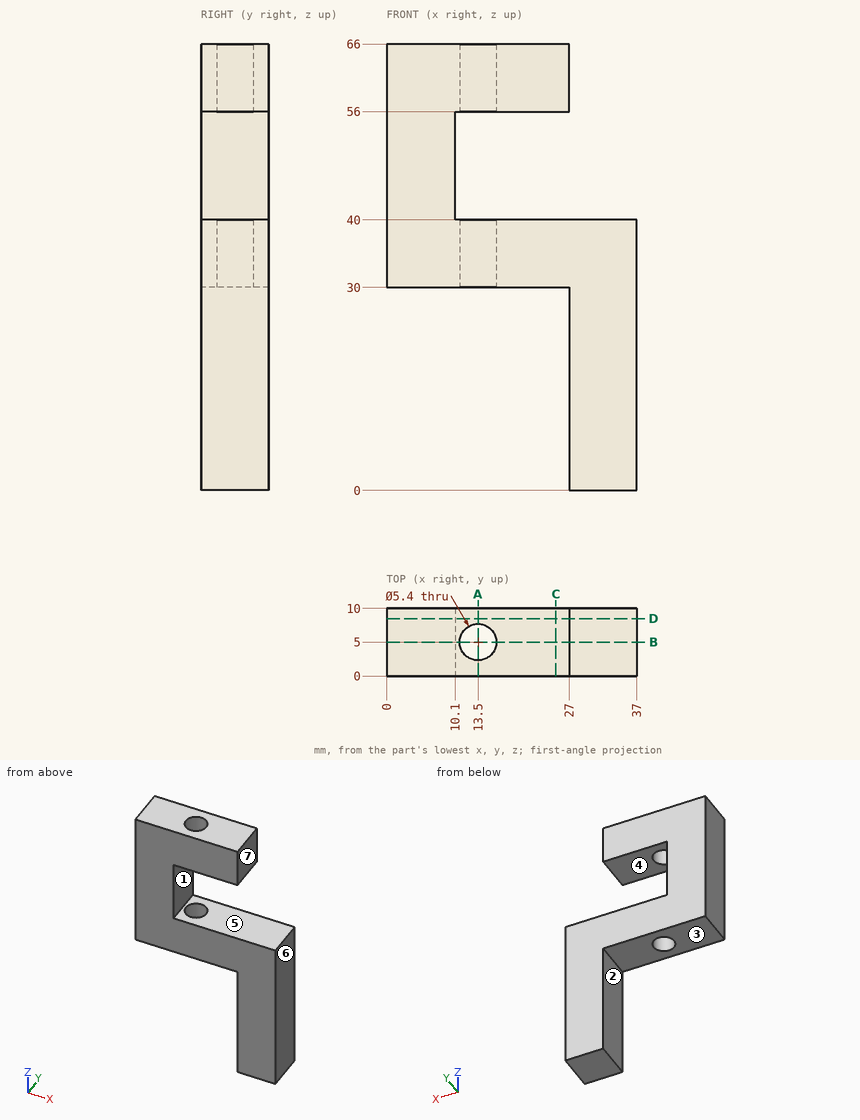
Design review of the part shown in the three views and the two pictorial views. Dimensions are in mm from the part's minimum x, y and z. A direction names the side the tool comes from. Coordinates: 2 decimals unless noted, no trailing zeros. Write each loop counter-clockwise with the first axis right and the second up, starting at its lowest first coordinate (ties: lowest second). Pieces come first, ordered by that corner, then holes.
1) We need section D-D on y = 8.5. State the section outline as (x, z) points.
2) We need section C-C on x = 25. State the section outline as (y, z) points.
3) We need section B-B on y = 5. State the section outline as (x, z) points, then the cut area to 3 significant figures.
4) The part is to be moulded in two halves that separate along Z. For the marked faces 1, 2, 3 and 4, say which applies: pulls with the +Z half, pulls with the -Z half, needs draft (parallel to the pull), parting line crosses it, or undercut.
5) To check wall thickness, follow probe 1 along Y at (x, z) = (13.5, 35.5); probe 2 along Z at (x, y) = (19.5, 8.5); probe 3 along X at (y, z) = (1.75, 19.5). State the ranges of each line that lie inside material, in increasing order.
6) Clearance check with flat-ended pins moving along their axes: pin 1 Ø3 at (x, y) = (13.5, 5) entering from -Z; pin 2 Ø1 at (x, y) = (7, 6) entering from -Z; pin 3 Ø1 at (y, z) = (5, 17.5) entering from -X. State where each tip first meets the part, or that it passes through.
7) We need section A-A on x = 13.5. State the section outline as (y, z) points.
8) Machinability: for the marked faces 5, 6 and 7, which of the approach directions +Z, -Z, +X, -X, +Y, -Y give a long, thin tool a straight path to every point of the face, cutting with its end or side? Answer none if there is none.
Answer list:
1. outline: (0, 30) - (27, 30) - (27, 0) - (37, 0) - (37, 40) - (10.1, 40) - (10.1, 56) - (27, 56) - (27, 66) - (0, 66) - close
2. outline: (0, 30) - (10, 30) - (10, 40) - (0, 40) - close; (0, 56) - (10, 56) - (10, 66) - (0, 66) - close
3. outline: (0, 30) - (10.8, 30) - (10.8, 40) - (10.1, 40) - (10.1, 56) - (10.8, 56) - (10.8, 66) - (0, 66) - close; (16.2, 30) - (27, 30) - (27, 0) - (37, 0) - (37, 40) - (16.2, 40) - close; (16.2, 56) - (27, 56) - (27, 66) - (16.2, 66) - close
3. area: 994 mm2
4. face 1: undercut
4. face 2: needs draft
4. face 3: pulls with the -Z half
4. face 4: undercut
5. probe 1: y = 0 to 2.3, 7.7 to 10
5. probe 2: z = 30 to 40, 56 to 66
5. probe 3: x = 27 to 37
6. pin 1: passes through
6. pin 2: stops at z = 30
6. pin 3: stops at x = 27
7. outline: (0, 30) - (2.3, 30) - (2.3, 40) - (0, 40) - close; (0, 56) - (2.3, 56) - (2.3, 66) - (0, 66) - close; (7.7, 30) - (10, 30) - (10, 40) - (7.7, 40) - close; (7.7, 56) - (10, 56) - (10, 66) - (7.7, 66) - close
8. face 5: +X, +Y, -Y
8. face 6: +Z, -Z, +X, +Y, -Y
8. face 7: +Z, +X, +Y, -Y
